Can you work these out from the model? Positions are in its coordinate system, mm. Face numbers are marked on the shaded views. A direction names the side the tool comes from. Give positions to 0.01 mm unless a question says otherwise; leave off trailing zeros. Order: outer loops, then holes, each group sorted by start corner. A loop starts at its lowest first (then second) coordinate and runs counter-clockwise, first axis right, second up. Notation, with made-up numbers: M 84.5,21.25 L 88.5,21.25 A26 ccw 88.5,45.25 Z; hole C 8.25,-5.5 d2. An arc over 180 degrees is marked long. One line per question, with ' | ' between items. Start each with the question number.
1) If we section it at A-A, the plane x = 0: Please give me the cut outline in (y, z).
2) Please list where these lines run through material, in increasing order: line 1 along X through (y, z) = (0, -59); line 2 along Y through (x, z) = (-14, 9); line 3 along Z through (x, y) = (-1, -26). Write a range as [from, to].
3) If we section it at B-B, the plane z = -73: Please give me the cut outline in (x, y).
4) If we section it at D-D, the plane z = -10: Please give me the cut outline in (x, y).
5) For the marked faces 1, 2 and 3, which set-ups out of +Z, -Z, +X, -X, +Y, -Y let a thin tool reach every point of the face, with its end or its side?
6) I'm going to push flat-ended pins straight in: pin 1 Ø17.5 at (x, z) = (71.5, -32.5) entering from -Y; pin 2 Ø4 at (x, y) = (-32, 7.5) entering from +Z; pin 3 Ø10 at (x, z) = (-46.5, -67.5) entering from +Y; pin 4 Ø5.5 at (x, y) = (-14, 14) entering from -Z. Where does each tip first touch, or does it pass through?
7) If we section it at C-C, the plane y = 14: Please give me the cut outline in (x, z), plus the area to 3 significant figures.
8) Thinking about a two-plate mould opening in X: for the marked faces 4, 5, 6 and 7, which applies, +X half, -X half, draft (parallel to the pull), parting line (faces both ways), or undercut?
```python
from build123d import *

# Parameters (mm, degrees)
F0_R     = 26.5
F0_R_2   = 3
F0_R_3   = 16.1
F1_DEPTH = 13
F2_DEPTH = 53
F3_SIZE  = 60
F5_DEPTH = 33


with BuildPart() as f1:
    # F0 (on Top) → F1 (new body)
    with BuildSketch(Plane.XY):
        with BuildLine():
            ThreePointArc((28.7271796725, -8.6457589641), (29.6800892028, -4.3694742147), (30, 0))
            ThreePointArc((30, 0), (29.6800892028, 4.3694742147), (28.7271796725, 8.6457589641))
            ThreePointArc((28.7271796725, 8.6457589641), (0, 30), (-28.7271796725, 8.6457589641))
            ThreePointArc((-28.7271796725, 8.6457589641), (-30, 0), (-28.7271796725, -8.6457589641))
            ThreePointArc((-28.7271796725, -8.6457589641), (0, -30), (28.7271796725, -8.6457589641))
        make_face()
        Circle(F0_R, mode=Mode.SUBTRACT)
        Circle(F0_R)
        with Locations((-14, -14)):
            Circle(F0_R_2, mode=Mode.SUBTRACT)
        with Locations((14, -14)):
            Circle(F0_R_2, mode=Mode.SUBTRACT)
        with Locations((-14, 14)):
            Circle(F0_R_2, mode=Mode.SUBTRACT)
        Circle(F0_R_3, mode=Mode.SUBTRACT)
        with Locations((14, 14)):
            Circle(F0_R_2, mode=Mode.SUBTRACT)
        with BuildLine():
            ThreePointArc((28.7271796725, 8.6457589641), (29.6800892028, 4.3694742147), (30, 0))
            ThreePointArc((30, 0), (29.6800892028, -4.3694742147), (28.7271796725, -8.6457589641))
            Line((28.7271796725, -8.6457589641), (87.8872200847, -8.6457589641))
            Line((87.8872200847, -8.6457589641), (87.8872200847, 8.6457589641))
            Line((87.8872200847, 8.6457589641), (28.7271796725, 8.6457589641))
        make_face()
        with BuildLine():
            ThreePointArc((-28.7271796725, -8.6457589641), (-30, 0), (-28.7271796725, 8.6457589641))
            Line((-28.7271796725, 8.6457589641), (-87.8872200847, 8.6457589641))
            Line((-87.8872200847, 8.6457589641), (-87.8872200847, -8.6457589641))
            Line((-87.8872200847, -8.6457589641), (-28.7271796725, -8.6457589641))
        make_face()
    extrude(amount=F1_DEPTH)

    # F0 (on Top) → F2 (join)
    with BuildSketch(Plane.XY):
        with BuildLine():
            ThreePointArc((28.7271796725, -8.6457589641), (29.6800892028, -4.3694742147), (30, 0))
            ThreePointArc((30, 0), (29.6800892028, 4.3694742147), (28.7271796725, 8.6457589641))
            ThreePointArc((28.7271796725, 8.6457589641), (0, 30), (-28.7271796725, 8.6457589641))
            ThreePointArc((-28.7271796725, 8.6457589641), (-30, 0), (-28.7271796725, -8.6457589641))
            ThreePointArc((-28.7271796725, -8.6457589641), (0, -30), (28.7271796725, -8.6457589641))
        make_face()
        Circle(F0_R, mode=Mode.SUBTRACT)
        with BuildLine():
            ThreePointArc((28.7271796725, 8.6457589641), (29.6800892028, 4.3694742147), (30, 0))
            ThreePointArc((30, 0), (29.6800892028, -4.3694742147), (28.7271796725, -8.6457589641))
            Line((28.7271796725, -8.6457589641), (87.8872200847, -8.6457589641))
            Line((87.8872200847, -8.6457589641), (87.8872200847, 8.6457589641))
            Line((87.8872200847, 8.6457589641), (28.7271796725, 8.6457589641))
        make_face()
        with BuildLine():
            ThreePointArc((-28.7271796725, -8.6457589641), (-30, 0), (-28.7271796725, 8.6457589641))
            Line((-28.7271796725, 8.6457589641), (-87.8872200847, 8.6457589641))
            Line((-87.8872200847, 8.6457589641), (-87.8872200847, -8.6457589641))
            Line((-87.8872200847, -8.6457589641), (-28.7271796725, -8.6457589641))
        make_face()
    extrude(amount=-F2_DEPTH)

    # F3
    f3_edges = [f1.edges().sort_by_distance(p)[0] for p in [
        (87.88722, 0, 13),
        (-87.88722, 0, 13),
    ]]
    chamfer(f3_edges, length=F3_SIZE)

    # F4 (on face) → F5 (join)
    with BuildSketch(Plane(origin=(0, 0, -53), x_dir=(1, 0, 0), z_dir=(0, 0, -1))):
        with BuildLine():
            ThreePointArc((-30.8099148317, -8.6457589641), (-32, 0), (-30.8099148317, 8.6457589641))
            Line((-30.8099148317, 8.6457589641), (-87.8872200847, 8.6457589641))
            Line((-87.8872200847, 8.6457589641), (-87.8872200847, -8.6457589641))
            Line((-87.8872200847, -8.6457589641), (-30.8099148317, -8.6457589641))
        make_face()
        with BuildLine():
            ThreePointArc((30.8099148317, 8.6457589641), (31.7010825889, 4.3636409904), (32, 0))
            ThreePointArc((32, 0), (31.7010825889, -4.3636409904), (30.8099148317, -8.6457589641))
            Line((30.8099148317, -8.6457589641), (87.8872200847, -8.6457589641))
            Line((87.8872200847, -8.6457589641), (87.8872200847, 8.6457589641))
            Line((87.8872200847, 8.6457589641), (30.8099148317, 8.6457589641))
        make_face()
    extrude(amount=F5_DEPTH)


solid = f1.part
```
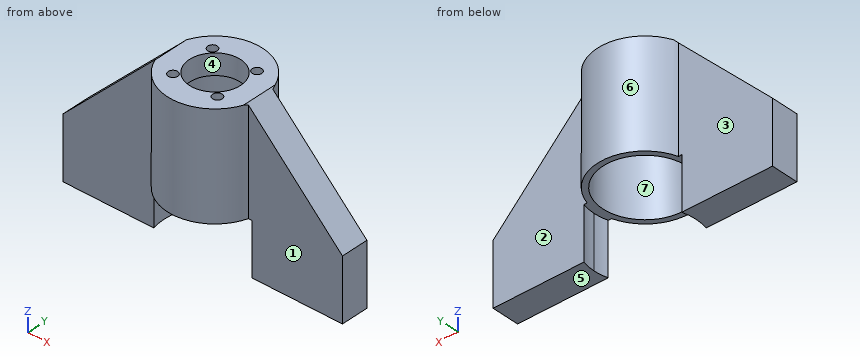
Results found:
1) outline: M -30,-53 L -26.5,-53 L -26.5,0 L -16.1,0 L -16.1,13 L -30,13 Z; M 16.1,0 L 26.5,0 L 26.5,-53 L 30,-53 L 30,13 L 16.1,13 Z
2) line 1: x = [-87.89, -32], [32, 87.89] | line 2: y = [-26.53, -17], [-11, -7.95], [7.95, 11], [17, 26.53] | line 3: z = [0, 13]
3) outline: M -87.89,-8.65 L -30.81,-8.65 A32 cw -30.81,8.65 L -87.89,8.65 Z; M 30.81,-8.65 L 87.89,-8.65 L 87.89,8.65 L 30.81,8.65 A32 cw Z
4) outline: M -50.89,-8.65 L -28.73,-8.65 A30 ccw 28.73,-8.65 L 50.89,-8.65 L 50.89,8.65 L 28.73,8.65 A30 ccw -28.73,8.65 L -50.89,8.65 Z; hole C 0,0 d53
5) face 1: +Z, -Z, +X, -Y | face 2: +Z, -Z, +X, +Y | face 3: +Z, -Z, -X, +Y
6) pin 1: stops at y = -8.65 | pin 2: stops at z = 10.89 | pin 3: stops at y = 8.65 | pin 4: passes through
7) outline: M -26.53,-53 L -22.5,-53 L -22.5,0 L -17,0 L -17,13 L -26.53,13 Z; M -11,0 L -7.95,0 L -7.95,13 L -11,13 Z; M 7.95,0 L 11,0 L 11,13 L 7.95,13 Z; M 17,0 L 22.5,0 L 22.5,-53 L 26.53,-53 L 26.53,13 L 17,13 Z | area: 755 mm²
8) face 4: undercut | face 5: draft | face 6: parting line | face 7: undercut
